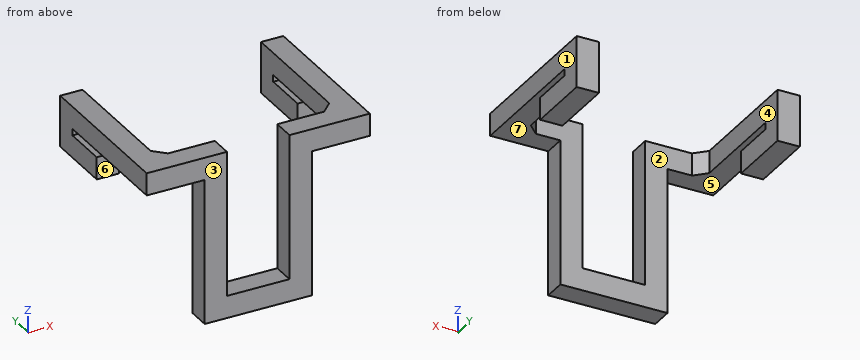
from build123d import *

# Parameters (mm, degrees)
BOSS_EXTRUDE1_DEPTH = 10
BOSS_EXTRUDE2_DEPTH = 10
BOSS_EXTRUDE3_DEPTH = 10
FILLET1_SIZE        = 5


with BuildPart() as part:
    # Sketch1 → Boss-Extrude1 (new body)
    with BuildSketch(Plane(origin=(0, 0, 0), x_dir=(0, 0, -1), z_dir=(1, 0, 0))):
        Polygon((0, 0), (0, 71), (23, 71), (23, 41), (13, 41), (13, 61), (10, 61), (10, 0), align=None)
    extrude(amount=BOSS_EXTRUDE1_DEPTH)

    # Sketch2 → Boss-Extrude2 (add)
    with BuildSketch(Plane(origin=(0, 0, 0), x_dir=(1, 0, 0), z_dir=(0, 1, 0))):
        Polygon((10, 0), (36, 0), (36, 65), (50, 65), (64, 65), (64, 0), (90, 0), (90, 10), (74, 10), (74, 75), (50, 75), (26, 75), (26, 10), (10, 10), align=None)
    extrude(amount=BOSS_EXTRUDE2_DEPTH)

    # Sketch3 → Boss-Extrude3 (add)
    with BuildSketch(Plane(origin=(90, 0, 0), x_dir=(0, 0, -1), z_dir=(1, 0, 0))):
        Polygon((0, 71), (0, 0), (10, 0), (10, 61), (13, 61), (13, 41), (23, 41), (23, 71), align=None)
    extrude(amount=BOSS_EXTRUDE3_DEPTH)

    # Fillet1
    fillet1_edges = [part.edges().sort_by_distance(p)[0] for p in [
        (10, 10, -5),
        (90, 10, -5),
    ]]
    chamfer(fillet1_edges, length=FILLET1_SIZE)


solid = part.part
Here's how the part is built. I have some questions about the finished solid (model axes, mm). Face numbers are marked on the shaded views. A direction names the side the tool comes from. Give positions to 0.01 mm unless a question says otherwise; leave off trailing zeros. Order: outer loops, then holes, each group sorted by start corner. A loop starts at its lowest first (then second) coordinate and runs counter-clockwise, first axis right, second up. Notation, with made-up numbers: (-24, 16.5) -> (11, 16.5) arc R30 ccw to (11, 55.5) -> close; hole circle Ø4 at (-31, 56.5). An arc over 180 degrees is marked (long way). Use a Markdown table: item, result. Add a question column.
Item 1: Imagine slicing it at D-D on z = -57. Please give me the cut outline in (x, y), plus the area to 3 significant figures.
Item 2: Imagine slicing it at B-B on z = -5. Please give me the cut outline in (x, y), plus the area to 4 significant figures.
Item 3: Will these pins go through, and if not, where does the flat tip stop? pin 1 (18.5 mm diameter, centred on y = 32, z = -16, fed in from +X); pin 2 (8 mm diameter, centred on x = 7.5, y = 53, fed in from -Z); pin 3 (1.5 mm diameter, centred on x = 95, z = -11, fed in from -Y); pin 4 (5 mm diameter, centred on x = 3.5, z = -17.5, fed in from -Y).
Item 4: Imagine slicing it at C-C on y = 64.5. Please give me the cut outline in (x, z), plus the area to 3 significant figures.
Item 5: If we mould it in two halves opening along X, with no side actions, what happens to the marked faces 1, 2 and 3? For each: pulls with the +X half, pulls with the -X half, needs draft (parallel to the pull), parting line crosses it, or undercut.
Item 6: For the marked faces 4, 5, 6 and 7, which set-ups out of +Z, -Z, +X, -X, +Y, -Y let a thin tool reach every point of the face, with its end or its side?
Item 7: I need wall thicknesses on line 1 (Y direction, x = 26, z = -3.5); line 2 (X direction, y = 46, z = -15); line 3 (Y direction, x = 85.5, z = -9.5). Which ranges of each line are inside material? Lowest first, please.
Item 8: Imagine slicing it at A-A on y = 57. Please give me the cut outline in (x, z), plus the area to 3 significant figures.
Data:
| question | item | result |
|---|---|---|
| 1 | outline | (26, 0) -> (36, 0) -> (36, 10) -> (26, 10) -> close; (64, 0) -> (74, 0) -> (74, 10) -> (64, 10) -> close |
| 1 | area | 200 mm² |
| 2 | outline | (0, 0) -> (36, 0) -> (36, 10) -> (15, 10) -> (10, 15) -> (10, 71) -> (0, 71) -> close; (64, 0) -> (100, 0) -> (100, 71) -> (90, 71) -> (90, 15) -> (85, 10) -> (64, 10) -> close |
| 2 | area | 1,965 mm² |
| 3 | pin 1 | stops at x = 100 |
| 3 | pin 2 | stops at z = -23 |
| 3 | pin 3 | stops at y = 61 |
| 3 | pin 4 | stops at y = 41 |
| 4 | outline | (0, -23) -> (10, -23) -> (10, 0) -> (0, 0) -> close; (90, -23) -> (100, -23) -> (100, 0) -> (90, 0) -> close |
| 4 | area | 460 mm² |
| 5 | face 1 | pulls with the +X half |
| 5 | face 2 | undercut |
| 5 | face 3 | needs draft |
| 6 | face 4 | +Z, -Z, +Y |
| 6 | face 5 | -X, -Y |
| 6 | face 6 | -Z, +X, -X, -Y |
| 6 | face 7 | +X, -Y |
| 7 | line 1 | y = 0 to 10 |
| 7 | line 2 | x = 0 to 10, 90 to 100 |
| 7 | line 3 | y = 0 to 10.5 |
| 8 | outline | (0, -23) -> (10, -23) -> (10, -13) -> (0, -13) -> close; (0, -10) -> (10, -10) -> (10, 0) -> (0, 0) -> close; (90, -23) -> (100, -23) -> (100, -13) -> (90, -13) -> close; (90, -10) -> (100, -10) -> (100, 0) -> (90, 0) -> close |
| 8 | area | 400 mm² |
